Build history of the part. All positions in model axes, mm. A direction names the side the tool comes from. Give positions to 0.01 mm unless a question says otherwise; leave off trailing zeros. Loops run counter-clockwise (first coordinate to the right, second up) from the corner with the lowest first, then second, coordinate; pieces in that order, holes last.
1) Wall check: line 1 (X direction, y = 29, z = 17.5); line 2 (Y direction, x = -28, z = 18.5); line 3 (Z direction, x = -16, y = 10). Give the ranges that are in metal, low to high.
2) 3-axis set-ups, long thin cutter, end or side, ignore diameter. For faces 4 (the flat face through (-11.152, 23, 18)), 5 (the cylindrical face through (-16.62, 6.35, 2.46)), 6 (the flat face through (-11.152, -12, 18)): which of +Z, -Z, +X, -X, +Y, -Y reach the whole face in a straight line?
3) Band-saw the part on A-A on z = 26.5. List the corners of the cut face in (x, y), then the cut area to 3 significant figures.
4) Band-saw the part on C-C on y = 31. List the corners of the cut face in (x, z), then the cut area to 3 significant figures.
5) Band-saw the part on D-D on z = 48. List the corners of the cut face in (x, y).
6) Band-saw the part on B-B on x = -28. List the corners of the cut face in (y, z).
7) Two-plate mould, pull along X, no slides. Class faces 1 (the flat face through (4, 8.241, 18)), 2 (the cylindrical face through (-10.44, 4.05, 43.64)), 3 (the cylindrical face through (-16.65, 5.61, 46.57)): +X half, -X half, draft (parallel to the pull), parting line (faces both ways), or undercut.
8) Flat gauge pins, fed straight in: P1, Ø24, axis at x = 9, z = 16, coming from the -Y side; P2, Ø9, axis at y = 25, z = 16, coming from the -X side; P3, Ø12, axis at y = 28.5, z = 11, coming from the +X side; P4, Ø8, axis at y = -16.5, z = 43, coming from the -X side. Where does each tip first touch, or does it go through?
```python
from build123d import *

# Parameters (mm, degrees)
SKETCH_1_W          = 5.5
SKETCH_1_H          = 30
SKETCH_1_W_2        = 30
SKETCH_1_H_2        = 5.5
EXTRUDE_1_DEPTH     = 36
SKETCH_5_R          = 3.75
EXTRUDE_3_DEPTH     = 15.5
SKETCH_6_R          = 2.85
CUT_EXTRUDE_1_DEPTH = 5
SKETCH_7_R          = 1.75
CUT_EXTRUDE_2_DEPTH = 52.5
SKETCH_8_R          = 2.75
CUT_EXTRUDE_3_DEPTH = 10


with BuildPart() as part:
    # 草圖1 → 填料-伸長1 (new body)
    with BuildSketch(Plane.XY):
        with Locations((-13.901604276, 23.24099723)):
            Rectangle(SKETCH_1_W, SKETCH_1_H)
        with Locations((-31.651604276, 5.49099723)):
            Rectangle(SKETCH_1_W_2, SKETCH_1_H_2)
        with Locations((-13.901604276, -12.25900277)):
            Rectangle(SKETCH_1_W, SKETCH_1_H)
        with Locations((3.848395724, 5.49099723)):
            Rectangle(SKETCH_1_W_2, SKETCH_1_H_2)
        with Locations((-13.901604276, 5.49099723)):
            Rectangle(SKETCH_1_W, SKETCH_1_H_2)
    extrude(amount=EXTRUDE_1_DEPTH)

    # 草圖5 → 填料-伸長3 (add)
    with BuildSketch(Plane.XY.offset(36)):
        with Locations((-13.901604276, 5.49099723)):
            Circle(SKETCH_5_R)
    extrude(amount=EXTRUDE_3_DEPTH)

    # 草圖6 → 除料-伸長1 (cut)
    with BuildSketch(Plane(origin=(0, 0, 0), x_dir=(-1, 0, 0), z_dir=(0, 0, -1))):
        with Locations((13.901604276, 5.49099723)):
            Circle(SKETCH_6_R)
    extrude(amount=-CUT_EXTRUDE_1_DEPTH, mode=Mode.SUBTRACT)

    # 草圖7 → 除料-伸長2 (cut, through all)
    with BuildSketch(Plane.XY.offset(51.5)):
        with Locations((-13.901604276, 5.49099723)):
            Circle(SKETCH_7_R)
    extrude(amount=-CUT_EXTRUDE_2_DEPTH, mode=Mode.SUBTRACT)

    # 草圖8 → 除料-伸長3 (cut)
    with BuildSketch(Plane.XY.offset(51.5)):
        with Locations((-13.901604276, 5.49099723)):
            Circle(SKETCH_8_R)
    extrude(amount=-CUT_EXTRUDE_3_DEPTH, mode=Mode.SUBTRACT)


solid = part.part
```
Findings below:
1. line 1: x = -16.65 to -11.15
1. line 2: y = 2.74 to 8.24
1. line 3: z = 0 to 36
2. face 4: +Z, -Z, +X, +Y
2. face 5: -Z
2. face 6: +Z, -Z, +X, -Y
3. outline: (-46.65, 2.74) - (-16.65, 2.74) - (-16.65, -27.26) - (-11.15, -27.26) - (-11.15, 2.74) - (18.85, 2.74) - (18.85, 8.24) - (-11.15, 8.24) - (-11.15, 38.24) - (-16.65, 38.24) - (-16.65, 8.24) - (-46.65, 8.24) - close; hole circle Ø3.5 at (-13.9, 5.49)
3. area: 681 mm2
4. outline: (-16.65, 0) - (-11.15, 0) - (-11.15, 36) - (-16.65, 36) - close
4. area: 198 mm2
5. outline: circle Ø7.5 at (-13.9, 5.49); hole circle Ø5.5 at (-13.9, 5.49)
6. outline: (2.74, 0) - (8.24, 0) - (8.24, 36) - (2.74, 36) - close
7. face 1: draft
7. face 2: parting line
7. face 3: undercut
8. P1: stops at y = 2.74
8. P2: stops at x = -16.65
8. P3: stops at x = -11.15
8. P4: passes through
